Check sheet for the modelled part. Datum: model origin and axes. Units: mm. A direction names the side the tool comes from. Give positions to 0.01 mm unless a question says otherwise; leave off trailing zeros. Order: outer loops, then holes, each group sorted by start corner. A loop starts at its lowest first (then second) coordinate and runs counter-clockwise, first axis right, second up. Notation, with made-up numbers: (-38, 14) - (-33, 14) arc R17 cw to (-33, 33) - close; hole circle Ø8 at (-28.75, 36.25). An arc over 180 degrees is marked (long way). Answer in a Markdown table with one row per item.
from build123d import *

# Parameters (mm, degrees)
SKETCH1_W               = 320
SKETCH1_H               = 200
SKETCH1_W_2             = 280
SKETCH1_H_2             = 160
BOSS_EXTRUDE1_DEPTH     = 20
SKETCH2_W               = 150
SKETCH2_H               = 200
CUT_EXTRUDE1_DEPTH      = 20
SKETCH3_W               = 20
SKETCH3_H               = 20
BOSS_EXTRUDE2_DEPTH     = 60
SKETCH4_W               = 10
SKETCH4_H               = 15
CUT_EXTRUDE2_DEPTH      = 20
SKETCH5_W               = 12
SKETCH5_H               = 12
CUT_EXTRUDE3_DEPTH      = 22
CUT_EXTRUDE5_DEPTH      = 275.40845468
CUT_EXTRUDE5_DEPTH_BACK = 275.40845468
SKETCH8_R               = 3
SKETCH10_R              = 3
CUT_EXTRUDE6_DEPTH      = 30
SKETCH11_W              = 14
SKETCH11_H              = 50
CUT_EXTRUDE7_DEPTH      = 6
SKETCH12_R              = 3
CUT_EXTRUDE8_DEPTH      = 20


with BuildPart() as part:
    # Sketch1 → Boss-Extrude1 (new body)
    with BuildSketch(Plane(origin=(0, 0, 0), x_dir=(1, 0, 0), z_dir=(0, 1, 0))):
        with Locations((160, 100)):
            Rectangle(SKETCH1_W, SKETCH1_H)
        with Locations((160, 100)):
            Rectangle(SKETCH1_W_2, SKETCH1_H_2, mode=Mode.SUBTRACT)
    extrude(amount=BOSS_EXTRUDE1_DEPTH)

    # Sketch2 → Cut-Extrude1 (cut)
    with BuildSketch(Plane(origin=(0, 20, 0), x_dir=(1, 0, 0), z_dir=(0, 1, 0))):
        with Locations((245, 100)):
            Rectangle(SKETCH2_W, SKETCH2_H)
    extrude(amount=-CUT_EXTRUDE1_DEPTH, mode=Mode.SUBTRACT)

    # Sketch3 → Boss-Extrude2 (add)
    with BuildSketch(Plane(origin=(0, 20, 0), x_dir=(1, 0, 0), z_dir=(0, 1, 0))):
        with Locations((10, 10)):
            Rectangle(SKETCH3_W, SKETCH3_H)
        with Locations((10, 190)):
            Rectangle(SKETCH3_W, SKETCH3_H)
    extrude(amount=BOSS_EXTRUDE2_DEPTH)

    # Sketch4 → Cut-Extrude2 (cut)
    with BuildSketch(Plane(origin=(0, 80, 0), x_dir=(1, 0, 0), z_dir=(0, 1, 0))):
        with Locations((10, 10)):
            Rectangle(SKETCH4_W, SKETCH4_H)
        with Locations((10, 190)):
            Rectangle(SKETCH4_W, SKETCH4_H)
    extrude(amount=-CUT_EXTRUDE2_DEPTH, mode=Mode.SUBTRACT)

    # Sketch5 → Cut-Extrude3 (cut)
    with BuildSketch(Plane(origin=(170, 0, 0), x_dir=(0, 0, -1), z_dir=(1, 0, 0))):
        with Locations((10, 10)):
            Rectangle(SKETCH5_W, SKETCH5_H)
        with Locations((190, 10)):
            Rectangle(SKETCH5_W, SKETCH5_H)
    extrude(amount=-CUT_EXTRUDE3_DEPTH, mode=Mode.SUBTRACT)

    # Sketch8 → Cut-Extrude5 (cut, two sides: drawn at the far end of the back side and taken through both)
    with BuildSketch(Plane(origin=(0, 0, -200), x_dir=(-1, 0, 0), z_dir=(0, 0, -1)).offset(-CUT_EXTRUDE5_DEPTH_BACK)):
        with Locations((-30, 10)):
            Circle(SKETCH8_R)
        with Locations((-160, 10)):
            Circle(SKETCH8_R)
        with Locations((-70, 10)):
            Circle(SKETCH8_R)
        with Locations((-130, 10)):
            Circle(SKETCH8_R)
    extrude(amount=CUT_EXTRUDE5_DEPTH + CUT_EXTRUDE5_DEPTH_BACK, mode=Mode.SUBTRACT)

    # Sketch10 → Cut-Extrude6 (cut)
    with BuildSketch(Plane.XZ):
        with Locations(Location((132.5, -10, 0), (0, 0, 270))):
            Circle(SKETCH10_R)
        with Locations(Location((85, -10, 0), (0, 0, 270))):
            Circle(SKETCH10_R)
        with Locations(Location((10, -100, 0), (0, 0, 270))):
            Circle(SKETCH10_R)
        with Locations(Location((132.5, -190, 0), (0, 0, 270))):
            Circle(SKETCH10_R)
        with Locations(Location((85, -190, 0), (0, 0, 270))):
            Circle(SKETCH10_R)
    extrude(amount=-CUT_EXTRUDE6_DEPTH, mode=Mode.SUBTRACT)

    # Sketch11 → Cut-Extrude7 (cut)
    with BuildSketch(Plane(origin=(20, 0, 0), x_dir=(0, 0, -1), z_dir=(1, 0, 0))):
        with Locations((7, 55)):
            Rectangle(SKETCH11_W, SKETCH11_H)
    extrude(amount=-CUT_EXTRUDE7_DEPTH, mode=Mode.SUBTRACT)

    # Sketch12 → Cut-Extrude8 (cut)
    with BuildSketch(Plane.ZY):
        with Locations((-133, 10)):
            Circle(SKETCH12_R)
        with Locations((-67, 10)):
            Circle(SKETCH12_R)
    extrude(amount=-CUT_EXTRUDE8_DEPTH, mode=Mode.SUBTRACT)


solid = part.part
(1) Cross-section at A-A, the plane y = 56.5. Record the cut outline in (x, z).
Geometry says:
| item | result |
|---|---|
| outline | (0, -200) - (20, -200) - (20, -180) - (0, -180) - close; (0, -20) - (20, -20) - (20, -14) - (14, -14) - (14, 0) - (0, 0) - close |
(2) Cross-section at B-B, the plane x = 70. Record the cut outline in (y, z).
Geometry says:
| item | result |
|---|---|
| outline | (0, -200) - (7, -200) - (7, -180) - (0, -180) - close; (0, -20) - (7, -20) - (7, 0) - (0, 0) - close; (13, -200) - (20, -200) - (20, -180) - (13, -180) - close; (13, -20) - (20, -20) - (20, 0) - (13, 0) - close |
(3) Gauge pin test, flat ends, axial feed: P1, Ø5.5, axis at x = 70, y = 10, coming from the -Z side; P2, Ø9.5, axis at x = 85, z = -190, coming from the -Y side; P3, Ø7.5, axis at y = 67, z = -7, coming from the +X side; P4, Ø22, axis at x = 131.5, z = -10.5, coming from the +Y side. Record the tip position at first contact, or that the pin passes through.
Geometry says:
| item | result |
|---|---|
| P1 | through |
| P2 | y = 0 |
| P3 | x = 5 |
| P4 | y = 20 |
(4) Thickness scan on L1, parallel to Z at x = 150.5, y = 8; L2, parallel to X at y = 5.25, z = -190; L3, parallel to Y at x = 70, z = -186. Record the ranges inside material, lowest first.
Geometry says:
| item | result |
|---|---|
| L1 | -200 to -196, -184 to -180, -20 to -16, -4 to 0 |
| L2 | 0 to 82, 88 to 129.5, 135.5 to 148 |
| L3 | 0 to 7, 13 to 20 |
(5) Mould release check, pull along Z, two halves, no side actions. Record for faces 5 (the flat face through (94, 20, -190)), 6 (the flat face through (10, 60, -190)), 7 (the flat face through (59, 19, -200)): pulls with the +Z half, pulls with the -Z half, needs draft (parallel to the pull), parting line crosses it, or undercut.
Geometry says:
| item | result |
|---|---|
| face 5 | needs draft |
| face 6 | undercut |
| face 7 | pulls with the -Z half |
(6) Access from +Z, -Z, +X, -X, +Y, -Y to the whole of each face (thin tool, end or side, straight path). Record for faces 1 (the flat face through (10, 60, -10)), 2 (the flat face through (9, 70, -2.5)), 3 (the flat face through (20, 42.9, -14.3)), 4 (the flat face through (17, 55, -14)).
Geometry says:
| item | result |
|---|---|
| face 1 | +Y |
| face 2 | +X, +Y |
| face 3 | +Z, -Z, +X, +Y |
| face 4 | +Z, +X, +Y |
(7) Cross-section at C-C, the plane z = -67. Record the cut outline in (x, y).
Geometry says:
| item | result |
|---|---|
| outline | (0, 0) - (20, 0) - (20, 7) - (0, 7) - close; (0, 13) - (20, 13) - (20, 20) - (0, 20) - close |
(8) Cross-section at D-D, the plane x = 48. Record the cut outline in (y, z), then the cut area to 3 significant figures.
Geometry says:
| item | result |
|---|---|
| outline | (0, -200) - (20, -200) - (20, -180) - (0, -180) - close; (0, -20) - (20, -20) - (20, 0) - (0, 0) - close |
| area | 800 mm² |
